```python
from build123d import *

# Parameters (mm, degrees)
SKETCH_1_R             = 62
SKETCH_1_R_2           = 60
EXTRUDE_1_DEPTH        = 3
EXTRUDE_START          = 6
SKETCH_2_R             = 48
EXTRUDE_2_DEPTH        = 6
FILLET_1_R             = 5
CHAMFER_1_SIZE         = 0.5
CHAMFER_2_SIZE         = 0.5
SKETCH_6_R             = 2.2
CUT_EXTRUDE_1_DEPTH    = 6
SKETCH_7_W             = 65
SKETCH_7_H             = 13.477482046
EXTRUDE_3_DEPTH        = 3
SKETCH_11_R            = 1.7
CUT_EXTRUDE_2_DEPTH    = 3
CHAMFER_3_SIZE         = 1
CHAMFER_4_SIZE         = 1
FILLET_2_R             = 3
CHAMFER_5_3_ANGLE      = 291.929687
SKETCH_12_R            = 4
CUT_EXTRUDE_3_DEPTH    = 3
CUT_EXTRUDE_4_DEPTH    = 2
CHAMFER_6_SIZE         = 1
HOLE_WIZARD_M3_1_D     = 2.5
HOLE_WIZARD_M3_1_DEPTH = 7.5
HOLE_WIZARD_M3_1_TIP   = 0.751075774
HOLE_WIZARD_M3_2_D     = 2.5
HOLE_WIZARD_M3_2_DEPTH = 7.5
HOLE_WIZARD_M3_2_TIP   = 0.751075774


with BuildPart() as part:
    # 草图1 → 凸台-拉伸1 (new body)
    with BuildSketch(Plane.XY):
        Circle(SKETCH_1_R)
        Circle(SKETCH_1_R_2, mode=Mode.SUBTRACT)
    extrude(amount=-EXTRUDE_1_DEPTH)

    # 草图2 → 凸台-拉伸2 (add)
    with BuildSketch(Plane.XY.offset(EXTRUDE_START)):
        with BuildLine():
            Line((-32.5, 63), (32.5, 63))
            Line((32.5, 63), (32.5, 52.79914772))
            ThreePointArc((32.5, 52.79914772), (0, -62), (-32.5, 52.79914772))
            Line((-32.5, 52.79914772), (-32.5, 63))
        make_face()
        Circle(SKETCH_2_R, mode=Mode.SUBTRACT)
    extrude(amount=-EXTRUDE_2_DEPTH)

    # 圆角1
    # the kernel refuses this fillet: 5 mm, written as the material it adds along each edge
    with BuildSketch(Plane(origin=(32.5, 52.79914772, 6), x_dir=(0.8403342947446245, -0.5420685132675156, 0), z_dir=(0, 0, -1))) as fillet_1_piece_1:
        with BuildLine():
            CenterArc((2.72541822, -4.998883971), FILLET_1_R, 91.210593649, 55.964843523)
            Line((-1.476253254, -2.288541405), (0, 0))
            ThreePointArc((0, 0), (1.309890927, -0.013838756), (2.619781855, 0))
        make_face()
    extrude(amount=6)
    with BuildSketch(Plane(origin=(-32.5, 52.79914772, 6), x_dir=(-0.840334294744627, -0.5420685132675117, 0), z_dir=(0, 0, -1))) as fillet_1_piece_2:
        with BuildLine():
            CenterArc((2.72541822, 4.998883971), FILLET_1_R, 212.824562828, 55.964843523)
            Line((-1.476253254, 2.288541405), (0, 0))
            ThreePointArc((0, 0), (1.309890927, 0.013838756), (2.619781855, 0))
        make_face()
    extrude(amount=6)

    # 倒角1
    chamfer_1_edges = [part.edges().sort_by_distance(p)[0] for p in [
        (-48, 0, 0),
        (-48, 0, 6),
        (-60, 0, -3),
    ]]
    chamfer(chamfer_1_edges, length=CHAMFER_1_SIZE)

    # 倒角2
    # the kernel refuses this chamfer: 0.5 mm, written as the material it takes off along each edge
    with BuildSketch(Plane(origin=(-32.5, 55.522517954, 0), x_dir=(0, 0, 1), z_dir=(0, 1, 0)), Plane(origin=(32.5, 64.285841494, 0), x_dir=(0, 0, 1), z_dir=(0, -1, 0))) as chamfer_2_piece_1:
        Polygon((CHAMFER_2_SIZE, 0), (0, CHAMFER_2_SIZE), (0, 0), align=None)
    extrude(amount=8.76332354, mode=Mode.SUBTRACT)
    with BuildSketch(Plane(origin=(37.5, 55.522517954, 0), x_dir=(-0.15613015555825177, -0.9877364904291813, 0), z_dir=(0.9877364904291813, -0.15613015555825177, 0))) as chamfer_2_piece_2_section:
        Polygon((5, -CHAMFER_2_SIZE), (5 + CHAMFER_2_SIZE, 0), (5, 0), align=None)
    chamfer_2_piece_2 = revolve(axis=Axis((37.5, 55.522517954, 0), (0, 0, -1)), revolution_arc=81.017652556, mode=Mode.PRIVATE)
    chamfer_2_piece_2 = chamfer_2_piece_2 - Plane(origin=(0, 0, 0), x_dir=(1, 0, 0), z_dir=(0, 0, 1)) * Cylinder(62, 22, mode=Mode.PRIVATE)
    add(chamfer_2_piece_2, mode=Mode.SUBTRACT)
    with BuildSketch(Plane(origin=(-37.5, 55.522517954, 0), x_dir=(1, 0, 0), z_dir=(0, 1, 0))) as chamfer_2_piece_3_section:
        Polygon((5, -CHAMFER_2_SIZE), (5 + CHAMFER_2_SIZE, 0), (5, 0), align=None)
    chamfer_2_piece_3 = revolve(axis=Axis((-37.5, 55.522517954, 0), (0, 0, -1)), revolution_arc=81.017652556, mode=Mode.PRIVATE)
    chamfer_2_piece_3 = chamfer_2_piece_3 - Plane(origin=(0, 0, 0), x_dir=(1, 0, 0), z_dir=(0, 0, 1)) * Cylinder(62, 22, mode=Mode.PRIVATE)
    add(chamfer_2_piece_3, mode=Mode.SUBTRACT)

    # 草图6 → 切除-拉伸1 (cut)
    with BuildSketch(Plane(origin=(0, 0, 0), x_dir=(-1, 0, 0), z_dir=(0, 0, -1))):
        with Locations((-42.877900702, 31.152618372)):
            Circle(SKETCH_6_R)
        with Locations((-53, 0)):
            Circle(SKETCH_6_R)
        with Locations((-42.877900702, -31.152618371)):
            Circle(SKETCH_6_R)
        with Locations((-16.377900702, -50.405995364)):
            Circle(SKETCH_6_R)
        with Locations((16.377900702, -50.405995364)):
            Circle(SKETCH_6_R)
        with Locations((42.877900702, -31.152618371)):
            Circle(SKETCH_6_R)
        with Locations((53, 0)):
            Circle(SKETCH_6_R)
        with Locations((42.877900702, 31.152618372)):
            Circle(SKETCH_6_R)
        with Locations((16.377900702, 50.405995364)):
            Circle(SKETCH_6_R)
        with Locations((-16.377900702, 50.405995364)):
            Circle(SKETCH_6_R)
    extrude(amount=-CUT_EXTRUDE_1_DEPTH, mode=Mode.SUBTRACT)

    # 草图7 → 凸台-拉伸3 (add)
    with BuildSketch(Plane.XY.offset(6)):
        with Locations((0, 62.261258977)):
            Rectangle(SKETCH_7_W, SKETCH_7_H)
    extrude(amount=EXTRUDE_3_DEPTH)

    # 草图11 → 切除-拉伸2 (cut)
    with BuildSketch(Plane.XY.offset(9)):
        with Locations((-29.5, 66)):
            Circle(SKETCH_11_R)
        with Locations((29.5, 66)):
            Circle(SKETCH_11_R)
    extrude(amount=-CUT_EXTRUDE_2_DEPTH, mode=Mode.SUBTRACT)

    # 倒角3
    chamfer_3_edges = [part.edges().sort_by_distance(p)[0] for p in [
        (0, 63, 0),
    ]]
    chamfer(chamfer_3_edges, length=CHAMFER_3_SIZE - 0.0001)  # a hair under: the kernel refuses the full size

    # 倒角4
    chamfer_4_edges = [part.edges().sort_by_distance(p)[0] for p in [
        (0, 55.522517954, 9),
    ]]
    chamfer(chamfer_4_edges, length=CHAMFER_4_SIZE)

    # 圆角2
    fillet_2_edges = [part.edges().sort_by_distance(p)[0] for p in [
        (-32.5, 69, 7.5),
        (32.5, 69, 7.5),
    ]]
    fillet(fillet_2_edges, radius=FILLET_2_R)

    # 倒角5: read off the stored shape, not the designer's step
    # 倒角5 outline → 倒角5 (revolve, cut)
    with BuildSketch(Plane(origin=(37.5, 55.522517954, 0), x_dir=(1, 0, 0), z_dir=(0, -1, 0))):
        Polygon((4.999998721, 9), (4.999998721, 4.999998721), (9, 9), align=None)
    revolve(axis=Axis((37.5, 55.522517954, 0), (0, 0, 1)), mode=Mode.SUBTRACT)

    # Chamfer 5 2 outline → Chamfer 5 2 (revolve, cut)
    with BuildSketch(Plane(origin=(-37.5, 55.522517954, 0), x_dir=(1, 0, 0), z_dir=(0, -1, 0))):
        Polygon((4.99999762, 9), (4.99999762, 4.99999762), (9, 9), align=None)
    revolve(axis=Axis((-37.5, 55.522517954, 0), (0, 0, 1)), mode=Mode.SUBTRACT)

    # Chamfer 5 3 outline → Chamfer 5 3 (revolve, cut)
    with BuildSketch(Plane(origin=(0, 0, 0), x_dir=(-0.5597014925373135, 0.8286942978273132, 0), z_dir=(0.8286942978273132, 0.5597014925373135, 0))):
        Polygon((62, 6), (61, 6), (62, 5), align=None)
    revolve(axis=Axis((0, 0, 0), (0, 0, 1)), revolution_arc=CHAMFER_5_3_ANGLE, mode=Mode.SUBTRACT)

    # 草图12 → 切除-拉伸3 (cut)
    with BuildSketch(Plane.XY.offset(6)):
        with Locations((-16.377900702, 50.405995364)):
            Circle(SKETCH_12_R)
        with Locations((16.377900702, 50.405995364)):
            Circle(SKETCH_12_R)
        with Locations((42.877900702, 31.152618372)):
            Circle(SKETCH_12_R)
        with Locations((53, 0)):
            Circle(SKETCH_12_R)
        with Locations((42.877900702, -31.152618371)):
            Circle(SKETCH_12_R)
        with Locations((16.377900702, -50.405995364)):
            Circle(SKETCH_12_R)
        with Locations((-16.377900702, -50.405995364)):
            Circle(SKETCH_12_R)
        with Locations((-42.877900702, -31.152618371)):
            Circle(SKETCH_12_R)
        with Locations((-53, 0)):
            Circle(SKETCH_12_R)
        with Locations((-42.877900702, 31.152618372)):
            Circle(SKETCH_12_R)
    extrude(amount=-CUT_EXTRUDE_3_DEPTH, mode=Mode.SUBTRACT)

    # 草图14 → 切除-拉伸4 (cut)
    with BuildSketch(Plane(origin=(0, 63, 0), x_dir=(1, 0, 0), z_dir=(0, 1, 0))):
        with BuildLine():
            ThreePointArc((-4.030108666, 3.809429698), (-11.733833556, 7.447967709), (-11.5, -1.068584287))
            ThreePointArc((-11.5, -1.068584287), (0, -4.15), (11.5, -1.068584287))
            ThreePointArc((11.5, -1.068584287), (11.733833556, 7.447967709), (4.030108666, 3.809429698))
            ThreePointArc((4.030108666, 3.809429698), (0, 5.85), (-4.030108666, 3.809429698))
        make_face()
    extrude(amount=-CUT_EXTRUDE_4_DEPTH, mode=Mode.SUBTRACT)

    # 倒角6
    # the kernel refuses this chamfer: 1 mm, written as the material it takes off along each edge
    with BuildSketch(Plane(origin=(18.80558547, 61, -3), x_dir=(0, -1, 0), z_dir=(-1, 0, 0))) as chamfer_6_piece_1:
        Polygon((CHAMFER_6_SIZE, 0), (0, CHAMFER_6_SIZE), (0, 0), align=None)
    extrude(amount=37.61117094, mode=Mode.SUBTRACT)
    with BuildSketch(Plane(origin=(-9, 63, -3.261542732), x_dir=(-0.874686173337968, 0, 0.48468969266055384), z_dir=(-0.48468969266055384, 0, -0.874686173337968))) as chamfer_6_piece_2:
        Polygon((5, -CHAMFER_6_SIZE), (5 + CHAMFER_6_SIZE, 0), (5, 0), align=None)
    revolve(axis=Axis((-9, 63, -3.261542732), (0, 1, 0)), revolution_arc=31.007856081, mode=Mode.SUBTRACT)
    with BuildSketch(Plane(origin=(9, 63, -3.261542732), x_dir=(0.49999999999998873, 0, 0.8660254037844451), z_dir=(-0.8660254037844451, 0, 0.49999999999998873))) as chamfer_6_piece_3:
        Polygon((5, -CHAMFER_6_SIZE), (5 + CHAMFER_6_SIZE, 0), (5, 0), align=None)
    revolve(axis=Axis((9, 63, -3.261542732), (0, 1, 0)), revolution_arc=31.007856081, mode=Mode.SUBTRACT)
    with BuildSketch(Plane(origin=(0, 63, -18.85), x_dir=(-0.500000000000001, 0, 0.8660254037844382), z_dir=(-0.8660254037844382, 0, -0.500000000000001))) as chamfer_6_piece_4:
        Polygon((23, -CHAMFER_6_SIZE), (23 + CHAMFER_6_SIZE, 0), (23, 0), align=None)
    revolve(axis=Axis((0, 63, -18.85), (0, 1, 0)), revolution_arc=60, mode=Mode.SUBTRACT)

    # M3 螺纹孔1
    with Locations(Plane.XY.offset(9)):
        with Locations((-25, 60), (25, 60)):
            Hole(HOLE_WIZARD_M3_1_D / 2, depth=HOLE_WIZARD_M3_1_DEPTH)
            with Locations((0, 0, -(HOLE_WIZARD_M3_1_DEPTH + HOLE_WIZARD_M3_1_TIP / 2))):  # 118° drill point
                Cone(0, HOLE_WIZARD_M3_1_D / 2, HOLE_WIZARD_M3_1_TIP, mode=Mode.SUBTRACT)

    # M3 螺纹孔2
    with Locations(Plane.XY.offset(6)):
        with Locations((0, -53)):
            Hole(HOLE_WIZARD_M3_2_D / 2, depth=HOLE_WIZARD_M3_2_DEPTH)
            with Locations((0, 0, -(HOLE_WIZARD_M3_2_DEPTH + HOLE_WIZARD_M3_2_TIP / 2))):  # 118° drill point
                Cone(0, HOLE_WIZARD_M3_2_D / 2, HOLE_WIZARD_M3_2_TIP, mode=Mode.SUBTRACT)


solid = part.part
```
CAD build for the part. Positions are in the model's coordinates, mm. A direction names the side the tool comes from. Round coordinates to 2 decimals unless told otherwise and drop trailing zeros. Answer in a Markdown table with one row per item. Add a question column.
Item 1: Saw through at A-A, the plane y = 0. Count the separate pieces of the cut face and the enclosed holes in it, then the cut area to 3 significant figures.
Item 2: Mould opens along Y. For faces 1 (the face through (0, 69, 7)), 2 (the face through (55.198, 0.097, 1.479)), 3 (the face through (0, 66, 6)) say: pulls with the +Y half, pulls with the -Y half, needs draft (parallel to the pull), parting line crosses it, or undercut.
Item 3: Which spindle directions (+Z, -Z, +X, -X, +Y, -Y) get a long thin tool onto all of the face, cutting with end or side? Do faces 4 (the face through (25, 60, 0)), 5 (the face through (23, -44, 6)), 6 (the face through (-49, 0, 0)), 7 (the face through (-25, 59, 0)), 8 (the face through (56.815, 1.201, 4.521)). Say none if no direction does.
Item 4: Drop flat-ended pins along their axis: pin 1 Ø7 at (x, y) = (16.38, -50.41) entering from +Z; pin 2 Ø9 at (x, y) = (16, -48.5) entering from +Z; pin 3 Ø6 at (y, z) = (31.5, 0.5) entering from +X; pin 4 Ø13 at (x, y) = (-16.38, 50.41) entering from +Z. Give the stop position or say it passes through.
Item 5: Drill centre lines: line 1 (X direction, y = -1, z = 4); line 2 (X direction, y = 48.5, z = 2.75); line 3 (Y direction, x = 37, z = 3.5). Where is each one in solid material? Low to high. Write a range as from..to.
Findings below:
| question | item | result |
|---|---|---|
| 1 | separate pieces | 4 |
| 1 | enclosed holes | 0 |
| 1 | area | 104 mm^2 |
| 2 | face 1 | pulls with the +Y half |
| 2 | face 2 | undercut |
| 2 | face 3 | needs draft |
| 3 | face 4 | -Z, +X, +Y |
| 3 | face 5 | +Z, +X, -X, -Y |
| 3 | face 6 | -Z |
| 3 | face 7 | -Z, -X, +Y |
| 3 | face 8 | +Z |
| 4 | pin 1 | stops at z = 3 |
| 4 | pin 2 | stops at z = 6 |
| 4 | pin 3 | stops at x = 55.06 |
| 4 | pin 4 | stops at z = 9 |
| 5 | line 1 | x = -61.99..-56.87, -49.13..-47.99, 47.99..49.13, 56.87..61.99 |
| 5 | line 2 | x = -38.62..-17.48, -15.28..15.28, 17.48..38.62 |
| 5 | line 3 | y = -49.75..-30.58, 30.58..49.75 |
